```python
from build123d import *

# Parameters (mm, degrees)
ESBO_O1_W                = 3
ESBO_O1_H                = 12
ESBO_O1_W_2              = 20
ESBO_O1_H_2              = 20
RESSALTO_EXTRUS_O1_DEPTH = 3


with BuildPart() as part:
    # Esboço1 → Ressalto-extrusão1 (new body)
    with BuildSketch(Plane.XY):
        Polygon((-31.216896784, 10.517052385), (-31.216896784, -1.482947615), (-34.216896784, -1.482947615), (-34.216896784, -13.482947615), (-31.216896784, -13.482947615), (-31.216896784, -25.482947615), (-31.216896784, -28.482947615), (-19.216896784, -28.482947615), (-19.216896784, -25.482947615), (-7.216896784, -25.482947615), (-7.216896784, -28.482947615), (4.783103216, -28.482947615), (24.783103216, -28.482947615), (24.783103216, -25.482947615), (36.783103216, -25.482947615), (36.783103216, -28.482947615), (48.783103216, -28.482947615), (48.783103216, -25.482947615), (48.783103216, -13.482947615), (51.783103216, -13.482947615), (51.783103216, -1.482947615), (48.783103216, -1.482947615), (48.783103216, 10.517052385), (51.783103216, 10.517052385), (51.783103216, 22.517052385), (48.783103216, 22.517052385), (48.783103216, 34.517052385), (48.783103216, 37.517052385), (36.783103216, 37.517052385), (36.783103216, 34.517052385), (24.783103216, 34.517052385), (24.783103216, 37.517052385), (-1.216896784, 37.517052385), (-7.216896784, 37.517052385), (-7.216896784, 34.517052385), (-19.216896784, 34.517052385), (-19.216896784, 37.517052385), (-31.216896784, 37.517052385), (-31.216896784, 34.517052385), (-31.216896784, 22.517052385), (-34.216896784, 22.517052385), (-34.216896784, 10.517052385), align=None)
        with Locations((8.783103216, 16.517052385)):
            Rectangle(ESBO_O1_W, ESBO_O1_H, mode=Mode.SUBTRACT)
        with Locations((8.783103216, -7.482947615)):
            Rectangle(ESBO_O1_W, ESBO_O1_H, mode=Mode.SUBTRACT)
        with Locations((36.783103216, 4.517052385)):
            Rectangle(ESBO_O1_W_2, ESBO_O1_H_2, mode=Mode.SUBTRACT)
    extrude(amount=RESSALTO_EXTRUS_O1_DEPTH)


solid = part.part
```
Verification items for the finished model (mm, model axes). A direction names the side the tool comes from. Coordinates: 2 decimals unless noted, no trailing zeros. Order: outer loops, then holes, each group sorted by start corner. A loop starts at its lowest first (then second) coordinate and runs counter-clockwise, first axis right, second up. Notation, with made-up numbers: (-28.5, 26.5) -> (4.5, 26.5) arc R19 ccw to (4.5, 51.5) -> close; hole circle Ø4 at (69, 78). An arc over 180 degrees is marked (long way). Answer as CSV lines item,"result". Start each with the question number.
1) Cross-section at A-A, the plane y = 7. Record the boundary of the cut face in (x, z).
2) Cross-section at C-C, the plane z = 2.4. Give the number of separate pieces and of enclosed holes in the cut face, then the cut area to 3 significant figures.
3) Release check for a two-part mould opening along Y. For faces 1 (the face through (50, 22.517, 1)), 2 (the face through (24.783, 36, 1)), 3 (the face through (37, -5.483, 1)) record: released by +Y, released by -Y, zero draft, split by the parting line, or undercut.
4) Cross-section at D-D, the plane x = -13.5. Record the boundary of the cut face in (y, z), then the cut area to 3 significant figures.
5) Material ranges on L1, parallel to Y at x = 8.5, z = 0.2; L2, parallel to X at y = 14, z = 2; L3, parallel to X at y = 21.5, z = 0.7, recorded low to high. Write a range as [from, to].
6) Gauge pin test, flat ends, axial feed: pin 1 Ø1.5 at (y, z) = (35.5, 1) entering from -X; pin 2 Ø0.9 at (y, z) = (-27, 1) entering from +X; pin 3 Ø1.5 at (x, z) = (50, 2) entering from -Y. Record the tip position at first contact, or that the pin passes through.
7) Set-up check for faces 4 (the face through (-31.217, 30, 1)), 5 (the face through (9, -13.483, 1)), 6 (the face through (50, 10.517, 1)), 7 (the face through (24.783, -27, 1)): record each of +Z, -Z, +X, -X, +Y, -Y from which the full face is reachable in a straight line by a thin tool's end or side.
8) Cross-section at B-B, the plane y = 16. Record the boundary of the cut face in (x, z).
Conclusion:
1,outline,"(-31.22, 0) -> (26.78, 0) -> (26.78, 3) -> (-31.22, 3) -> close; (46.78, 0) -> (48.78, 0) -> (48.78, 3) -> (46.78, 3) -> close"
2,separate pieces,"1"
2,enclosed holes,"3"
2,area,"4,810 mm²"
3,face 1,"released by +Y"
3,face 2,"zero draft"
3,face 3,"undercut"
4,outline,"(-25.48, 0) -> (34.52, 0) -> (34.52, 3) -> (-25.48, 3) -> close"
4,area,"180 mm²"
5,L1,"y = [-28.48, -13.48], [-1.48, 10.52], [22.52, 37.52]"
5,L2,"x = [-34.22, 7.28], [10.28, 26.78], [46.78, 51.78]"
5,L3,"x = [-34.22, 7.28], [10.28, 51.78]"
6,pin 1,"stops at x = -31.22"
6,pin 2,"stops at x = 48.78"
6,pin 3,"stops at y = -13.48"
7,face 4,"+Z, -Z, -X, +Y"
7,face 5,"+Z, -Z"
7,face 6,"+Z, -Z, +X"
7,face 7,"+Z, -Z, -Y"
8,outline,"(-34.22, 0) -> (7.28, 0) -> (7.28, 3) -> (-34.22, 3) -> close; (10.28, 0) -> (51.78, 0) -> (51.78, 3) -> (10.28, 3) -> close"
